The model under review builds one solid part; all positions refer to its coordinate system, in mm. A direction names the side the tool comes from. Round coordinates to 2 decimals unless told otherwise and drop trailing zeros. Loops run counter-clockwise (first coordinate to the right, second up) from the corner with the lowest first, then second, coordinate; pieces in that order, holes last. Notation, with made-up numbers: M -39.5,-10 L -29.5,-10 A17 cw -29.5,21 Z; hole C 17.5,-22.75 d2. An arc over 180 degrees is marked long. Answer as a JSON object with one key per item and string values. Group by question number.
Item 1: Consider section B-B (y = 0). Give the boundary of the cut face in (x, z), and give its area (3 significant figures).
Item 2: Consider section D-D (z = 0.5). Give the boundary of the cut face in (x, y), and give its area (3 significant figures).
Item 3: Consider section C-C (z = 8). Give the boundary of the cut face in (x, y) (3 decimals), and give its area (4 significant figures).
Item 4: Consider section A-A (z = 9.5). Give the boundary of the cut face in (x, y) (3 decimals), and give its area (3 significant figures).
Item 5: To check wall thickness, follow line 1 (Y direction, x = 0, z = 3.45); line 2 (Y direction, x = 0, z = 3.25); line 3 (Z direction, x = -0.25, y = 16.5) (3 decimals). State the ranges of each line that lie inside material, in increasing order.
Item 6: The part is to be moulded in two halves that separate along Y. For faces 4 (the face through (-5.5, 20.175, 7.3)), 5 (the face through (-4.95, 20, 7)), 6 (the face through (5, 17, 2.675)), say which applies: +Y half, -Y half, draft (parallel to the pull), parting line (faces both ways), or undercut.
Item 7: Tool access review of faces 1 (the face through (5, 17, 2.325)), 2 (the face through (5.492, 19.577, 2.91)), 3 (the face through (-7, -2, 4)): name each direction out of +Z, -Z, +X, -X, +Y, -Y from which nothing blocks a thin tool from reaching the whole face with its end or side.
Item 8: Insertion check: P1, Ø1.8, axis at x = -6, y = 17.5, coming from the -Z side (3 decimals); P2, Ø5, axis at x = 2, y = -2.5, coming from the +Z side; P3, Ø2, axis at x = 7.5, y = -0.5, coming from the +Z side; P4, Ø2.5, axis at x = 6, y = 16.5, coming from the -Z side. Each pin has a flat end and moves straight along its axis. Give the tip position at first contact, or say it passes through.
```python
from build123d import *

# Parameters (mm, degrees)
SKETCH_1_W          = 16
SKETCH_1_H          = 21
SKETCH_1_R          = 1.75
EXTRUDE_1_DEPTH     = 5
EXTRUDE_1_2_DEPTH   = 16
CUT_EXTRUDE_1_DEPTH = 16
SKETCH_4_W          = 3.81913455
SKETCH_4_H          = 4
CUT_EXTRUDE_2_DEPTH = 2.5
SKETCH_5_R          = 0.1
CUT_EXTRUDE_3_DEPTH = 2


with BuildPart() as part:
    # Эскиз1 → Extrude 1 (new body)
    with BuildSketch(Plane.XY):
        with Locations((0, 5)):
            Rectangle(SKETCH_1_W, SKETCH_1_H)
        Circle(SKETCH_1_R, mode=Mode.SUBTRACT)
    extrude(amount=EXTRUDE_1_DEPTH)

    # Эскиз2 → Extrude 1 2 (add)
    with BuildSketch(Plane.ZY.offset(8)):
        with BuildLine():
            Line((2.675, 15.5), (2.675, 19))
            ThreePointArc((2.675, 19), (2.916636906, 19.583363094), (3.5, 19.825))
            Line((3.5, 19.825), (11, 19.825))
            Line((11, 19.825), (11, 20.175))
            Line((11, 20.175), (3.5, 20.175))
            ThreePointArc((3.5, 20.175), (2.669149532, 19.830850468), (2.325, 19))
            Line((2.325, 19), (2.325, 15.5))
            Line((2.325, 15.5), (2.675, 15.5))
        make_face()
    extrude(amount=-EXTRUDE_1_2_DEPTH)

    # Эскиз3 → Вырез-Вытянуть1 (cut)
    with BuildSketch(Plane(origin=(0, 0, 2.325), x_dir=(-1, 0, 0), z_dir=(0, 0, -1))):
        Polygon((-1.75, 15.5), (-1.75, 18.5), (-0.55, 19), (-0.55, 20.937907948), (-4.95, 20.937907948), (-4.95, 19), (-4.4, 18.622085888), (-4.4, 15.5), align=None)
        Polygon((0.55, 19), (0.55, 20.937907948), (4.95, 20.937907948), (4.95, 19), (4.4, 18.622085888), (4.4, 15.5), (1.75, 15.5), (1.75, 18.5), align=None)
        Polygon((-6.05, 19), (-6.05, 20.937907948), (-9.320905805, 20.937907948), (-9.320905805, 15.5), (-6.6, 15.5), (-6.6, 18.622085888), align=None)
        Polygon((6.05, 19), (6.05, 20.937907948), (9.499807758, 20.937907948), (9.499807758, 15.5), (6.6, 15.5), (6.6, 18.622085888), align=None)
    extrude(amount=-CUT_EXTRUDE_1_DEPTH, mode=Mode.SUBTRACT)

    # Эскиз4 → Вырез-Вытянуть2 (cut)
    with BuildSketch(Plane(origin=(0, 0, 5), x_dir=(-1, 0, 0), z_dir=(0, 0, -1))):
        with Locations((7.909567275, 0)):
            Rectangle(SKETCH_4_W, SKETCH_4_H)
        with Locations((-7.909567275, 0)):
            Rectangle(SKETCH_4_W, SKETCH_4_H)
    extrude(amount=CUT_EXTRUDE_2_DEPTH, mode=Mode.SUBTRACT)

    # Эскиз5 → Вырез-Вытянуть3 (cut)
    with BuildSketch(Plane.XY.offset(11)):
        with Locations((0, 20)):
            Circle(SKETCH_5_R)
    extrude(amount=-CUT_EXTRUDE_3_DEPTH, mode=Mode.SUBTRACT)


solid = part.part
```
Geometry results:
{
 "1": {"outline": "M -8,0 L -1.75,0 L -1.75,5 L -6,5 L -6,2.5 L -8,2.5 Z; M 1.75,0 L 8,0 L 8,2.5 L 6,2.5 L 6,5 L 1.75,5 Z", "area": "52.5 mm^2"},
 "2": {"outline": "M -8,-5.5 L 8,-5.5 L 8,15.5 L -8,15.5 Z; hole C 0,0 d3.5", "area": "326 mm^2"},
 "3": {"outline": "M -6.05,19.825 L -4.95,19.825 L -4.95,20.175 L -6.05,20.175 Z; M -0.55,19.825 L 0.55,19.825 L 0.55,20.175 L -0.55,20.175 Z; M 4.95,19.825 L 6.05,19.825 L 6.05,20.175 L 4.95,20.175 Z", "area": "1.155 mm^2"},
 "4": {"outline": "M -6.05,19.825 L -4.95,19.825 L -4.95,20.175 L -6.05,20.175 Z; M -0.55,19.825 L 0.55,19.825 L 0.55,20.175 L -0.55,20.175 Z; M 4.95,19.825 L 6.05,19.825 L 6.05,20.175 L 4.95,20.175 Z; hole C 0,20 d0.2", "area": "1.12 mm^2"},
 "5": {"line 1": "y = -5.5 to -1.75, 1.75 to 15.5, 19.82 to 20.17", "line 2": "y = -5.5 to -1.75, 1.75 to 15.5, 19.79 to 20.15", "line 3": "z = 2.325 to 2.675"},
 "6": {"face 4": "+Y half", "face 5": "draft", "face 6": "undercut"},
 "7": {"face 1": "-Z, +X, -X, +Y", "face 2": "+Z, +X, -X", "face 3": "+Z, -X"},
 "8": {"P1": "stops at z = 2.325", "P2": "stops at z = 5", "P3": "stops at z = 2.5", "P4": "stops at z = 0"}
}
